```python
from build123d import *

# Parameters (mm, degrees)
F0_R     = 27.011072
F0_R_2   = 11.036563
F1_DEPTH = 1
F2_DEPTH = 5


with BuildPart() as f1:
    # F0 (on Front) → F1 (new body)
    with BuildSketch(Plane.XZ):
        Circle(F0_R)
        Circle(F0_R_2, mode=Mode.SUBTRACT)
    extrude(amount=F1_DEPTH)

    # F0 (on Front) → F2 (join)
    with BuildSketch(Plane.XZ):
        with BuildLine():
            ThreePointArc((29.67797, -4.699063), (29.95511, -2.356792), (30.04768, 0))
            ThreePointArc((30.04768, 0), (29.95511, 2.356792), (29.67797, 4.699063))
            ThreePointArc((29.67797, 4.699063), (29.121812, 7.401566), (28.320102, 10.04166))
            ThreePointArc((28.320102, 10.04166), (27.333629, 12.479416), (26.137785, 14.821582))
            ThreePointArc((26.137785, 14.821582), (0, 30.04768), (-26.137785, 14.821582))
            ThreePointArc((-26.137785, 14.821582), (-27.333629, 12.479416), (-28.320102, 10.04166))
            ThreePointArc((-28.320102, 10.04166), (-29.121812, 7.401566), (-29.67797, 4.699063))
            ThreePointArc((-29.67797, 4.699063), (-30.04768, 0), (-29.67797, -4.699063))
            ThreePointArc((-29.67797, -4.699063), (-29.121812, -7.401566), (-28.320102, -10.04166))
            ThreePointArc((-28.320102, -10.04166), (-27.333629, -12.479416), (-26.137785, -14.821582))
            ThreePointArc((-26.137785, -14.821582), (0, -30.04768), (26.137785, -14.821582))
            ThreePointArc((26.137785, -14.821582), (27.333629, -12.479416), (28.320102, -10.04166))
            ThreePointArc((28.320102, -10.04166), (29.121812, -7.401566), (29.67797, -4.699063))
        make_face()
        Circle(F0_R, mode=Mode.SUBTRACT)
        Circle(F0_R_2)
        with BuildLine():
            ThreePointArc((26.137785, 14.821582), (27.333629, 12.479416), (28.320102, 10.04166))
            Line((28.320102, 10.04166), (50.103527, 10.04166))
            ThreePointArc((50.103527, 10.04166), (52.493488, 12.431621), (50.103527, 14.821582))
            Line((50.103527, 14.821582), (26.137785, 14.821582))
        make_face()
        with BuildLine():
            ThreePointArc((29.67797, 4.699063), (29.95511, 2.356792), (30.04768, 0))
            ThreePointArc((30.04768, 0), (29.95511, -2.356792), (29.67797, -4.699063))
            Line((29.67797, -4.699063), (59.423488, -4.699063))
            ThreePointArc((59.423488, -4.699063), (64.122551, 0), (59.423488, 4.699063))
            Line((59.423488, 4.699063), (29.67797, 4.699063))
        make_face()
        with BuildLine():
            Line((50.103527, -10.04166), (28.320102, -10.04166))
            ThreePointArc((28.320102, -10.04166), (27.333629, -12.479416), (26.137785, -14.821582))
            Line((26.137785, -14.821582), (50.103527, -14.821582))
            ThreePointArc((50.103527, -14.821582), (52.493488, -12.431621), (50.103527, -10.04166))
        make_face()
        with BuildLine():
            Line((-50.103527, -14.821582), (-26.137785, -14.821582))
            ThreePointArc((-26.137785, -14.821582), (-27.333629, -12.479416), (-28.320102, -10.04166))
            Line((-28.320102, -10.04166), (-50.103527, -10.04166))
            ThreePointArc((-50.103527, -10.04166), (-52.493488, -12.431621), (-50.103527, -14.821582))
        make_face()
        with BuildLine():
            ThreePointArc((-29.67797, -4.699063), (-30.04768, 0), (-29.67797, 4.699063))
            Line((-29.67797, 4.699063), (-59.423488, 4.699063))
            ThreePointArc((-59.423488, 4.699063), (-64.122551, 0), (-59.423488, -4.699063))
            Line((-59.423488, -4.699063), (-29.67797, -4.699063))
        make_face()
        with BuildLine():
            ThreePointArc((-28.320102, 10.04166), (-27.333629, 12.479416), (-26.137785, 14.821582))
            Line((-26.137785, 14.821582), (-50.103527, 14.821582))
            ThreePointArc((-50.103527, 14.821582), (-52.493488, 12.431621), (-50.103527, 10.04166))
            Line((-50.103527, 10.04166), (-28.320102, 10.04166))
        make_face()
    extrude(amount=F2_DEPTH)


solid = f1.part
```
For this review, take the finished solid that the model builds, in its own axes (mm). A direction names the side the tool comes from. Round coordinates to 2 decimals unless told otherwise and drop trailing zeros. Write each loop counter-clockwise with the first axis right and the second up, starting at its lowest first coordinate (ties: lowest second). Pieces come first, ordered by that corner, then holes. Notation, with made-up numbers: M 86.5,13 L 107.5,13 A30 cw 107.5,42 Z; hole C 57,-8.75 d2. An arc over 180 degrees is marked long. One line per item, written item: value. Start each with the question number.
(1) The part is to be moulded in two halves that separate along Z. For faces 4 (the flat face through (19, -5, -20)), 5 (the cylindrical face through (64.12, -2.46, -0.1)), 6 (the cylindrical face through (-29.11, -2.46, 7.44)), say which applies: released by +Z, released by -Z, zero draft, split by the parting line, or undercut.
(2) We need section C-C (z = 0). Give the boundary of the cut face in (x, y).
(3) We need section B-B (x = 0). Give the boundary of the cut face in (y, z), and give its area (3 significant figures).
(4) Insertion check: pin 1 (1.5 mm diameter, centred on x = 44, y = -2, fed in from +Z); pin 2 (1.5 mm diameter, centred on x = 37.5, y = -3, fed in from -Z); pin 3 (2 mm diameter, centred on x = -14, y = -1, fed in from +Z). Each pin has a flat end and moves straight along its axis. Give the tip position at first contact, or say it passes through.
(5) Wall thickness on line 1 (Z direction, x = -45.5, y = -0.35); line 2 (Z direction, x = 0, y = -3.7); line 3 (X direction, y = -2.15, z = 2): over which ranges is each line inside the solid? List them lowest first.
(6) Machinability: for faces 1 (the flat face through (45, -2, 4.699)), 2 (the flat face through (0, -1, -12)), 3 (the flat face through (-38, -2, 14.822)), which of the approach directions +Z, -Z, +X, -X, +Y, -Y give a long, thin tool a straight path to every point of the face, cutting with its end or side? Answer none if there is none.
(7) We need section D-D (z = -17.5). Give the boundary of the cut face in (x, y), and give its area (3 significant figures).
(8) We need section A-A (y = -3.3). Give the boundary of the cut face in (x, z).
Result:
1. face 4: zero draft
1. face 5: split by the parting line
1. face 6: undercut
2. outline: M -64.12,-5 L -27.01,-5 L -27.01,-1 L -11.04,-1 L -11.04,-5 L 11.04,-5 L 11.04,-1 L 27.01,-1 L 27.01,-5 L 64.12,-5 L 64.12,0 L -64.12,0 Z
3. outline: M -5,-30.05 L 0,-30.05 L 0,30.05 L -5,30.05 L -5,27.01 L -1,27.01 L -1,11.04 L -5,11.04 L -5,-11.04 L -1,-11.04 L -1,-27.01 L -5,-27.01 Z
3. area: 173 mm²
4. pin 1: z = 14.82
4. pin 2: z = -14.82
4. pin 3: z = 27.09
5. line 1: -14.82 to -10.04, -4.7 to 4.7, 10.04 to 14.82
5. line 2: -30.05 to -27.01, -11.04 to 11.04, 27.01 to 30.05
5. line 3: -63.68 to -26.94, -10.85 to 10.85, 26.94 to 63.68
6. face 1: +X, +Y, -Y
6. face 2: -Y
6. face 3: +Z, -X, +Y, -Y
7. outline: M -24.43,-5 L -20.58,-5 L -20.58,-1 L 20.58,-1 L 20.58,-5 L 24.43,-5 L 24.43,0 L -24.43,0 Z
7. area: 79.7 mm²
8. outline: M -59.42,-4.7 L -29.68,-4.7 A30.05 ccw -28.32,-10.04 L -50.1,-10.04 A2.39 ccw -50.1,-14.82 L -26.14,-14.82 A30.05 ccw 26.14,-14.82 L 50.1,-14.82 A2.39 ccw 50.1,-10.04 L 28.32,-10.04 A30.05 ccw 29.68,-4.7 L 59.42,-4.7 A4.7 ccw 59.42,4.7 L 29.68,4.7 A30.05 ccw 28.32,10.04 L 50.1,10.04 A2.39 ccw 50.1,14.82 L 26.14,14.82 A30.05 ccw -26.14,14.82 L -50.1,14.82 A2.39 ccw -50.1,10.04 L -28.32,10.04 A30.05 ccw -29.68,4.7 L -59.42,4.7 A4.7 ccw Z; C 0,0 d22.07; hole C 0,0 d54.02
